Geometry: final body of the model. Coordinates: model frame, mm. Face numbers are marked on the shaded views. A direction names the side the tool comes from. Coordinates: 2 decimals unless noted, no trailing zeros. Loops run counter-clockwise (first coordinate to the right, second up) from the corner with the lowest first, then second, coordinate; pieces in that order, holes last. Notation, with made-up numbers: (18, -2) -> (26, -2) arc R16 ccw to (26, 29) -> close; hole circle Ø3 at (35.25, -17.5). An arc over 180 degrees is marked (long way). One line per item, written item: value. Start each with the question number.
from build123d import *

# Parameters (mm, degrees)
SKETCH_W        = 30
SKETCH_H        = 15
PAD_DEPTH       = 1
SKETCH001_W     = 13.5
SKETCH001_H     = 15
SKETCH001_W_2   = 11.5
PAD001_DEPTH    = 2.5
SKETCH002_W     = 9.5
SKETCH002_H     = 11
SKETCH002_W_2   = 7.5
POCKET_DEPTH    = 2.5
SKETCH003_W     = 27.6
SKETCH003_H     = 12.6
SKETCH003_W_2   = 26
SKETCH003_H_2   = 11
PAD002_DEPTH    = 2
SKETCH004_W     = 5
SKETCH004_H     = 1.2
POCKET001_DEPTH = 13.801
SKETCH005_R     = 2
SKETCH005_W     = 5.7
SKETCH005_H     = 8.5
POCKET002_DEPTH = 5.501
SKETCH006_W     = 1
SKETCH006_H     = 6
PAD003_DEPTH    = 5.3
SKETCH007_W     = 7
SKETCH007_H     = 1
PAD004_DEPTH    = 2


with BuildPart() as part:
    # Sketch → Pad (new body)
    with BuildSketch(Plane.XY):
        Rectangle(SKETCH_W, SKETCH_H)
    extrude(amount=PAD_DEPTH)

    # Sketch001 (on Face6 of Pad) → Pad001 (join)
    with BuildSketch(Plane.XY.offset(1)):
        with Locations((-8.25, 0)):
            Rectangle(SKETCH001_W, SKETCH001_H)
        with Locations((9.25, 0)):
            Rectangle(SKETCH001_W_2, SKETCH001_H)
    extrude(amount=PAD001_DEPTH)

    # Sketch002 (on Face1 of Pad001) → Pocket (cut)
    with BuildSketch(Plane(origin=(0, 0, 0), x_dir=(1, 0, 0), z_dir=(0, 0, -1))):
        with Locations((-8.25, 0)):
            Rectangle(SKETCH002_W, SKETCH002_H)
        with Locations((9.25, 0)):
            Rectangle(SKETCH002_W_2, SKETCH002_H)
    extrude(amount=-POCKET_DEPTH, mode=Mode.SUBTRACT)

    # Sketch003 (on Face1 of Pocket) → Pad002 (join)
    with BuildSketch(Plane(origin=(0, 0, 0), x_dir=(1, 0, 0), z_dir=(0, 0, -1))):
        Rectangle(SKETCH003_W, SKETCH003_H)
        Rectangle(SKETCH003_W_2, SKETCH003_H_2, mode=Mode.SUBTRACT)
    extrude(amount=PAD002_DEPTH)

    # Sketch004 (on Face13 of Pad002) → Pocket001 (cut, through all)
    with BuildSketch(Plane.XZ.offset(6.3)):
        with Locations((0, -0.6)):
            Rectangle(SKETCH004_W, SKETCH004_H)
    extrude(amount=-POCKET001_DEPTH, mode=Mode.SUBTRACT)

    # Sketch005 (on Face16 of Pocket001) → Pocket002 (cut, through all)
    with BuildSketch(Plane.XY.offset(3.5)):
        with Locations((1, 0)):
            Circle(SKETCH005_R)
        with Locations((8, 0)):
            Rectangle(SKETCH005_W, SKETCH005_H)
        Polygon((-11.25, 6.5), (-11.25, 2), (-12.45, 2), (-12.45, -2), (-11.25, -2), (-11.25, -6.5), (-4.75, -6.5), (-4.75, 6.5), align=None)
    extrude(amount=-POCKET002_DEPTH, mode=Mode.SUBTRACT)

    # Sketch006 (on Face60 of Pocket002) → Pad003 (join)
    with BuildSketch(Plane(origin=(0, 0, 0), x_dir=(1, 0, 0), z_dir=(0, 0, -1))):
        with Locations((-3, 0)):
            Rectangle(SKETCH006_W, SKETCH006_H)
    extrude(amount=PAD003_DEPTH)

    # Sketch007 (on Face39 of Pad003) → Pad004 (join)
    with BuildSketch(Plane(origin=(0, 0, 0), x_dir=(1, 0, 0), z_dir=(0, 0, -1))):
        with Locations((0, 5)):
            Rectangle(SKETCH007_W, SKETCH007_H)
        with Locations((0, -5)):
            Rectangle(SKETCH007_W, SKETCH007_H)
    extrude(amount=PAD004_DEPTH)


solid = part.part
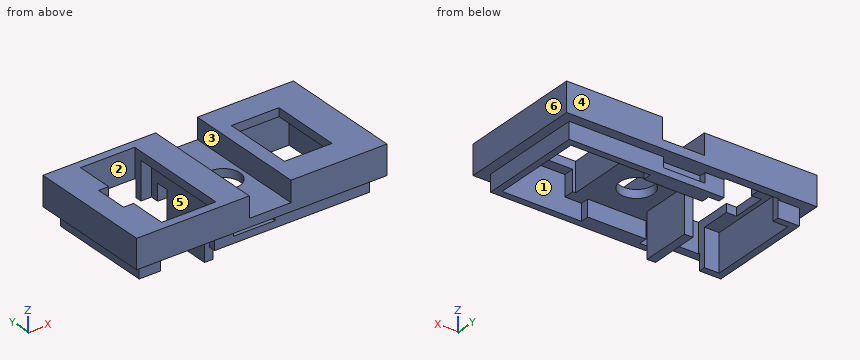
1. Line query: L1, parallel to X at y = 5.25, z = 2; L2, parallel to X at y = -3.75, z = 3.25; L3, parallel to Y at x = 1, z = 0.45. Output: solid intervals per line, ascending. Write a range as [from, to].
2. Section C-C on x = 1. Return the cut outline in (y, z).
3. Section D-D on y = 0. Count the separate pieces of the cut face and the enclosed holes in it, plus the area to 3 significant figures.
4. Draft query along X for the marked faces 4, 5 and 6. Return one class per face: released by +X, released by -X, zero draft, split by the parting line, or undercut.
5. Set-up query: the marked faces 1, 2 and 3. Return all of +Z, -Z, +X, -X, +Y, -Y with unobstructed straight access to the full face (end or side cutting, diameter ignored); none if empty.
6. Section B-B on z = 2. Return the cut outline in (x, y), plus the area to 3 significant figures.
7. Section A-A on y = 2.5. Return the cut outline in (x, z).
8. Pin query (flat end, axial travel): pin 1 Ø1.9 at (x, y) = (-12, 0) entering from -Z; pin 2 Ø0.6 at (y, z) = (6, -0.5) entering from -X; pin 3 Ø1.1 at (y, z) = (5, -1) entering from +X; pin 4 Ø4 at (x, z) = (-12, -1) entering from -Y. Return the tip coordinate at first contact, or that it passes through.
Checks:
1. L1: [-15, -13], [-3.5, -1.5], [3.5, 5.5], [13, 15]
1. L2: [-15, -11.25], [-4.75, -1.5], [3.5, 5.15], [10.85, 15]
1. L3: [-7.5, -2], [2, 7.5]
2. outline: (-7.5, 0) -> (-5.5, 0) -> (-5.5, -1.2) -> (-6.3, -1.2) -> (-6.3, -2) -> (-4.5, -2) -> (-4.5, 0) -> (-2, 0) -> (-2, 1) -> (-7.5, 1) -> close; (2, 0) -> (4.5, 0) -> (4.5, -2) -> (6.3, -2) -> (6.3, -1.2) -> (5.5, -1.2) -> (5.5, 0) -> (7.5, 0) -> (7.5, 1) -> (2, 1) -> close
3. separate pieces: 4
3. enclosed holes: 0
3. area: 40.2 mm²
4. face 4: zero draft
4. face 5: undercut
4. face 6: released by +X
5. face 1: -Z
5. face 2: +Z, -Z
5. face 3: +Z, +Y, -Y
6. outline: (-15, -7.5) -> (-1.5, -7.5) -> (-1.5, 7.5) -> (-15, 7.5) -> close; (3.5, -7.5) -> (15, -7.5) -> (15, 7.5) -> (3.5, 7.5) -> close; hole (-13, -5.5) -> (-11.25, -5.5) -> (-11.25, -6.5) -> (-4.75, -6.5) -> (-4.75, -5.5) -> (-3.5, -5.5) -> (-3.5, 5.5) -> (-4.75, 5.5) -> (-4.75, 6.5) -> (-11.25, 6.5) -> (-11.25, 5.5) -> (-13, 5.5) -> close; hole (5.15, -4.25) -> (5.5, -4.25) -> (5.5, -5.5) -> (13, -5.5) -> (13, 5.5) -> (5.5, 5.5) -> (5.5, 4.25) -> (5.15, 4.25) -> close
6. area: 172 mm²
7. outline: (-15, 0) -> (-13.8, 0) -> (-13.8, -2) -> (-13, -2) -> (-13, 2.5) -> (-11.25, 2.5) -> (-11.25, 3.5) -> (-15, 3.5) -> close; (-4.75, 2.5) -> (-3.5, 2.5) -> (-3.5, -5.3) -> (-2.5, -5.3) -> (-2.5, 0) -> (5.15, 0) -> (5.15, 3.5) -> (3.5, 3.5) -> (3.5, 1) -> (-1.5, 1) -> (-1.5, 3.5) -> (-4.75, 3.5) -> close; (10.85, 2.5) -> (13, 2.5) -> (13, -2) -> (13.8, -2) -> (13.8, 0) -> (15, 0) -> (15, 3.5) -> (10.85, 3.5) -> close
8. pin 1: z = 2.5
8. pin 2: x = -13.8
8. pin 3: x = 13.8
8. pin 4: y = -7.5
